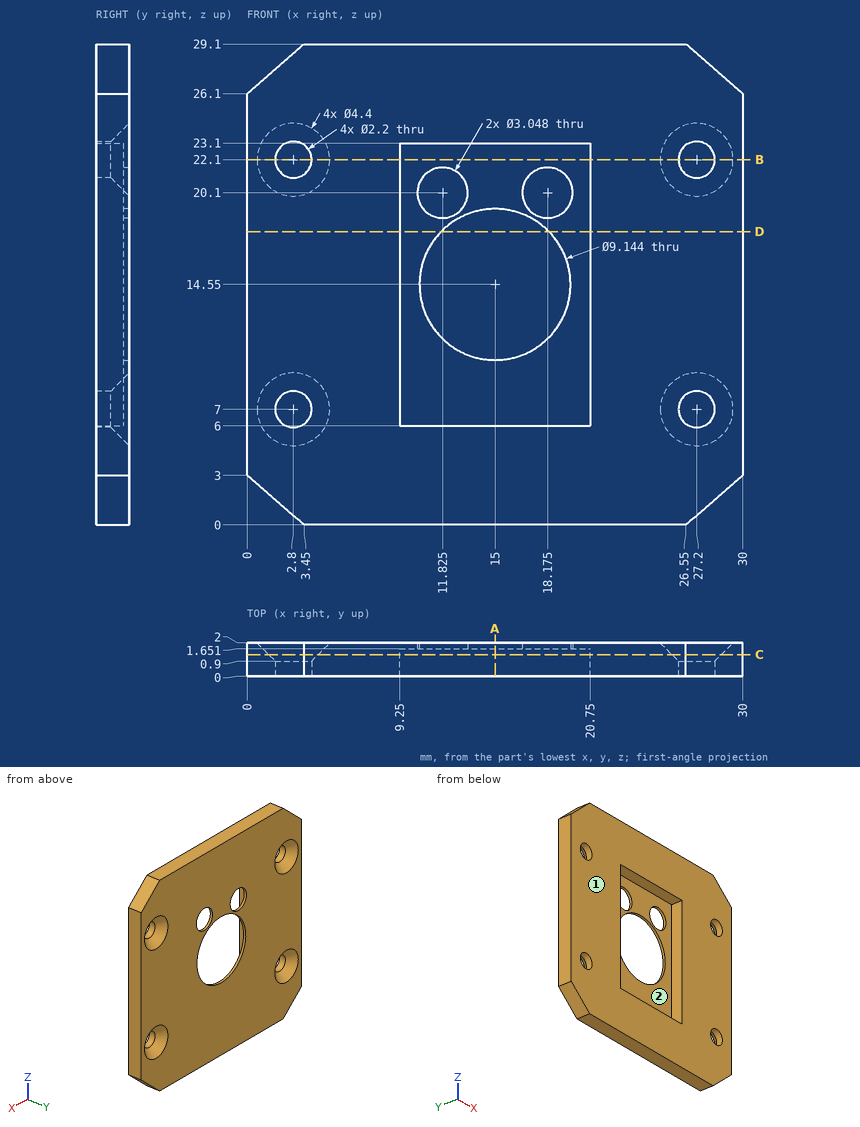
Job drawing, mm, ordinate dimensions from the low corner. One solid piece. Give positions to 0.01 mm unless a question says otherwise; leave off trailing zeros. Write each loop counter-clockwise with the first axis right and the second up, starting at its lowest first coordinate (ties: lowest second). Pieces come first, ordered by that corner, then holes. Notation, with made-up numbers: (84, 8) - (112, 8) arc R10 ccw to (112, 20) - close; hole circle Ø7 at (69, 85.25). An arc over 180 degrees is marked (long way). Use one line per item in the form item = value. Start each with the question number.
1. Probe line 1 (X direction, y = 0.2, z = 22.1); line 2 (Z direction, x = 20, y = 0.65); line 3 (X direction, y = 0.8, z = 13.75). List the from-to ranges inside material, lowest first. Write a range as [from, to].
2. Band-saw the part on D-D on z = 17.75. Write the cut outline in (x, y), plus the area to 3 significant figures.
3. Band-saw the part on B-B on z = 22.1. Write the cut outline in (x, y), plus the area to 3 significant figures.
4. Drop flat-ended pins along their axis: pin 1 Ø3.5 at (x, z) = (2.8, 7) entering from +Y; pin 2 Ø3.5 at (x, z) = (17.5, 16) entering from -Y; pin 3 Ø1.3 at (x, z) = (27.2, 22.1) entering from +Y. Give the stop position or say it passes through.
5. Band-saw the part on C-C on y = 1.3. Write the cut outline in (x, z), plus the area to 3 significant figures.
6. Two-plate mould, pull along X, no slides. Class the marked faces 1 and 2: released by +X, released by -X, zero draft, split by the parting line, or undercut.
7. Band-saw the part on A-A on x = 15. Write the cut outline in (y, z).
Conclusion:
q1.line_1 = [0, 1.7], [3.9, 9.25], [20.75, 26.1], [28.3, 30]
q1.line_2 = [0, 6], [23.1, 29.1]
q1.line_3 = [0, 9.25], [20.75, 30]
q2.outline = (0, 0) - (9.25, 0) - (9.25, 1.65) - (11.73, 1.65) - (11.73, 2) - (0, 2) - close; (18.27, 1.65) - (20.75, 1.65) - (20.75, 0) - (30, 0) - (30, 2) - (18.27, 2) - close
q2.area = 38.7 mm²
q3.outline = (0, 0) - (1.7, 0) - (1.7, 0.9) - (0.6, 2) - (0, 2) - close; (3.9, 0) - (9.25, 0) - (9.25, 1.65) - (20.75, 1.65) - (20.75, 0) - (26.1, 0) - (26.1, 0.9) - (25, 2) - (5, 2) - (3.9, 0.9) - close; (28.3, 0) - (30, 0) - (30, 2) - (29.4, 2) - (28.3, 0.9) - close
q3.area = 29.8 mm²
q4.pin_1 = 1.55
q4.pin_2 = 1.65
q4.pin_3 = through
q5.outline = (0, 3) - (3.45, 0) - (26.55, 0) - (30, 3) - (30, 26.1) - (26.55, 29.1) - (3.45, 29.1) - (0, 26.1) - close; hole circle Ø3 at (2.8, 7); hole circle Ø3 at (2.8, 22.1); hole (9.25, 6) - (20.75, 6) - (20.75, 23.1) - (9.25, 23.1) - close; hole circle Ø3 at (27.2, 7); hole circle Ø3 at (27.2, 22.1)
q5.area = 627 mm²
q6.face_1 = zero draft
q6.face_2 = undercut
q7.outline = (0, 0) - (2, 0) - (2, 9.98) - (1.65, 9.98) - (1.65, 6) - (0, 6) - close; (0, 23.1) - (1.65, 23.1) - (1.65, 19.12) - (2, 19.12) - (2, 29.1) - (0, 29.1) - close
